Build history of the part. All positions in model axes, mm. A direction names the side the tool comes from. Round coordinates to 2 decimals unless told otherwise and drop trailing zeros. Write each loop counter-clockwise with the first axis right and the second up, starting at its lowest first coordinate (ties: lowest second). Pieces come first, ordered by that corner, then holes. Notation, with made-up numbers: M -21,38 L 14,38 A27 cw 14,63 Z; hole C -20.5,-26.5 d6. An arc over 180 degrees is marked long. Write item = value, one per line. Start each with the question number.
Q1. Band-saw the part on A-A on x = -50. Write the cut outline in (y, z).
Q2. Band-saw the part on C-C on x = -11. Write the cut outline in (y, z), plus the area to 3 significant figures.
Q3. Band-saw the part on D-D on x = 73. Write the cut outline in (y, z).
Q4. Pull direction X, two halves, no side cores. Call faces 4 (the flat face through (-21, 4, 2)), 5 (the cylindrical face through (-72.95, 4.37, 1.52)), 6 (the flat face through (50, -6.5, 2)): released by +X, released by -X, zero draft, split by the parting line, or undercut.
Q5. Probe L1, parallel to Y at x = 80, z = 1.25; L2, parallel to X at y = 0.25, z = 1.35; L3, parallel to Y at x = -50, z = 2.05. List the from-to ranges inside material, lowest first.
Q6. Band-saw the part on B-B on z = 1.15. State how many separate pieces and enclosed holes the cut face has, plus the area to 3 significant figures.
Q7. Drop flat-ended pins along their axis: P1, Ø1.5, axis at x = 19.5, z = 2, coming from the -Y side; P2, Ø1.5, axis at x = 60, z = 2, coming from the +Y side; P3, Ø1.5, axis at y = -4.5, z = 1.5, coming from the +X side. Give the stop position or say it passes through.
Q8. Tool access for faces 1 (the flat face through (22, 4, 2)), 2 (the flat face through (22, -4, 2)), 3 (the cylindrical face through (-77.504, 0.11, 1.479)): list every direction of +Z, -Z, +X, -X, +Y, -Y with a clear straight run to the whole face (end or side of a thin tool).
```python
from build123d import *

# Parameters (mm, degrees)
SKETCH1_R           = 1.5
BOSS_EXTRUDE1_DEPTH = 3
SKETCH3_W           = 1.998076211
SKETCH3_H           = 3
FILLET1_R           = 48
BOSS_EXTRUDE3_DEPTH = 3
SKETCH8_R           = 1.4
CUT_EXTRUDE3_DEPTH  = 4
SKETCH9_R           = 4
BOSS_EXTRUDE6_DEPTH = 3


with BuildPart() as part:
    # Sketch1 → Boss-Extrude1 (new body)
    with BuildSketch(Plane.XY):
        with BuildLine():
            Line((-76.080816412, -4), (76.080816412, -4))
            ThreePointArc((76.080816412, -4), (85.6, 0), (76.080816412, 4))
            Line((76.080816412, 4), (-76.080816412, 4))
            ThreePointArc((-76.080816412, 4), (-85.6, 0), (-76.080816412, -4))
        make_face()
        with Locations((-80, 0)):
            Circle(SKETCH1_R, mode=Mode.SUBTRACT)
        with Locations((80, 0)):
            Circle(SKETCH1_R, mode=Mode.SUBTRACT)
    extrude(amount=BOSS_EXTRUDE1_DEPTH)

    # Sketch3 → Cut-Revolve1 (revolve, cut)
    with BuildSketch(Plane(origin=(0, 0, 0), x_dir=(1, 0, 0), z_dir=(0, 1, 0))):
        with Locations((81.499038106, -1.5)):
            Rectangle(SKETCH3_W, SKETCH3_H)
    cut_revolve1 = revolve(axis=Axis((80, 0, 0), (0, 0, 1)), mode=Mode.SUBTRACT)

    # Mirror1: Cut-Revolve1 across plane
    add(cut_revolve1.mirror(Plane(origin=(0, 0, 0), x_dir=(0, 0, 1), z_dir=(1, 0, 0))), mode=Mode.SUBTRACT)

    # Fillet1
    fillet1_edges = [part.edges().sort_by_distance(p)[0] for p in [
        (76.080816412, -4, 1.5),
        (-76.080816412, -4, 1.5),
        (-76.080816412, 4, 1.5),
        (76.080816412, 4, 1.5),
    ]]
    fillet(fillet1_edges, radius=FILLET1_R)

    # Sketch4 → Boss-Extrude3 (add, through all)
    with BuildSketch(Plane.XY.offset(3)):
        with BuildLine():
            Line((0, -4.4), (0.107106781, -4.292893219))
            ThreePointArc((0.107106781, -4.292893219), (0.43153013, -4.076120467), (0.814213562, -4))
            Line((0.814213562, -4), (4.4, -4))
            Line((4.4, -4), (4.4, 4))
            Line((4.4, 4), (0.814213562, 4))
            ThreePointArc((0.814213562, 4), (0.43153013, 4.076120467), (0.107106781, 4.292893219))
            Line((0.107106781, 4.292893219), (0, 4.4))
            Line((0, 4.4), (-0.107106781, 4.292893219))
            ThreePointArc((-0.107106781, 4.292893219), (-0.43153013, 4.076120467), (-0.814213562, 4))
            Line((-0.814213562, 4), (-4.4, 4))
            Line((-4.4, 4), (-4.4, -4))
            Line((-4.4, -4), (-0.814213562, -4))
            ThreePointArc((-0.814213562, -4), (-0.43153013, -4.076120467), (-0.107106781, -4.292893219))
            Line((-0.107106781, -4.292893219), (0, -4.4))
        make_face()
    extrude(amount=-BOSS_EXTRUDE3_DEPTH)

    # Sketch8 → Cut-Extrude3 (cut, through all)
    with BuildSketch(Plane.XY.offset(3)):
        with Locations((-50, 0)):
            Circle(SKETCH8_R)
        Polygon((51.732050808, 0), (50.866025404, 1.5), (49.133974596, 1.5), (48.267949192, 0), (49.133974596, -1.5), (50.866025404, -1.5), align=None)
    extrude(amount=-CUT_EXTRUDE3_DEPTH, mode=Mode.SUBTRACT)

    # Sketch9 → Boss-Extrude6 (add, through all)
    with BuildSketch(Plane.XY.offset(3)):
        with BuildLine():
            Line((38, -4), (43.07179677, -4))
            ThreePointArc((43.07179677, -4), (44.57179677, -4.401923789), (45.669872981, -5.5))
            Line((45.669872981, -5.5), (46.24722325, -6.5))
            Line((46.24722325, -6.5), (53.75277675, -6.5))
            Line((53.75277675, -6.5), (54.330127019, -5.5))
            ThreePointArc((54.330127019, -5.5), (55.42820323, -4.401923789), (56.92820323, -4))
            Line((56.92820323, -4), (62, -4))
            Line((62, -4), (62, 4))
            Line((62, 4), (56.92820323, 4))
            ThreePointArc((56.92820323, 4), (55.42820323, 4.401923789), (54.330127019, 5.5))
            Line((54.330127019, 5.5), (53.75277675, 6.5))
            Line((53.75277675, 6.5), (46.24722325, 6.5))
            Line((46.24722325, 6.5), (45.669872981, 5.5))
            ThreePointArc((45.669872981, 5.5), (44.57179677, 4.401923789), (43.07179677, 4))
            Line((43.07179677, 4), (38, 4))
            Line((38, 4), (38, -4))
        make_face()
        with Locations((50, 0)):
            Circle(SKETCH9_R, mode=Mode.SUBTRACT)
        with BuildLine():
            Line((-58.732124598, -4), (-62, -4))
            Line((-62, -4), (-62, 4))
            Line((-62, 4), (-58.732124598, 4))
            ThreePointArc((-58.732124598, 4), (-55.979715185, 4.386247225), (-53.439927872, 5.515151515))
            ThreePointArc((-53.439927872, 5.515151515), (-50, 6.5), (-46.560072128, 5.515151515))
            ThreePointArc((-46.560072128, 5.515151515), (-44.020284815, 4.386247225), (-41.267875402, 4))
            Line((-41.267875402, 4), (-38, 4))
            Line((-38, 4), (-38, -4))
            Line((-38, -4), (-41.267875402, -4))
            ThreePointArc((-41.267875402, -4), (-44.020284815, -4.386247225), (-46.560072128, -5.515151515))
            ThreePointArc((-46.560072128, -5.515151515), (-50, -6.5), (-53.439927872, -5.515151515))
            ThreePointArc((-53.439927872, -5.515151515), (-55.979715185, -4.386247225), (-58.732124598, -4))
        make_face()
        with Locations((-50, 0)):
            Circle(SKETCH9_R, mode=Mode.SUBTRACT)
    extrude(amount=-BOSS_EXTRUDE6_DEPTH)


solid = part.part
```
Conclusion:
q1.outline = M -6.5,0 L -1.4,0 L -1.4,3 L -6.5,3 Z; M 1.4,0 L 6.5,0 L 6.5,3 L 1.4,3 Z
q2.outline = M -4,0 L 4,0 L 4,3 L -4,3 Z
q2.area = 24.0 mm^2
q3.outline = M -4.38,0 L 4.38,0 L 4.38,3 L -4.38,3 Z
q4.face_4 = undercut
q4.face_5 = undercut
q4.face_6 = zero draft
q5.L1 = -5.6 to -2.5, 2.5 to 5.6
q5.L2 = -85.59 to -82.49, -77.51 to -51.38, -48.62 to 48.41, 51.59 to 77.51, 82.49 to 85.59
q5.L3 = -6.5 to -1.4, 1.4 to 6.5
q6.separate_pieces = 1
q6.enclosed_holes = 4
q6.area = 1,440 mm^2
q7.P1 = -4
q7.P2 = 4
q7.P3 = 84.16
q8.face_1 = +Z, -Z, +Y
q8.face_2 = +Z, -Z, -Y
q8.face_3 = +Z, -Z
